Part print with two shaded views. Sizes in mm from the minimum x, y, z corner. A direction names the side the tool comes from. Round coordinates to 2 decimals unless told otherwise and drop trailing zeros. Loops run counter-clockwise (first coordinate to the right, second up) from the corner with the lowest first, then second, coordinate; pieces in that order, holes last. Notation, with made-up numbers: M 80,7.5 L 87,7.5 A20 cw 87,39.5 Z; hole C -39.5,10.5 d8. An arc over 180 degrees is marked long. Answer as CSV lines item,"result". Start each with the question number.
Item 1: Drop flat-ended pins along their axis: pin 1 Ø0.7 at (y, z) = (6.5, 2) entering from -X; pin 2 Ø3 at (x, z) = (4.5, 5.5) entering from -Y; pin 3 Ø0.8 at (x, y) = (11.5, 0.5) entering from +Z. Give the stop position or say it passes through.
Item 2: Band-saw the part on A-A (x = 12.25). Give the cut face in (y, z), and give its area (3 significant figures).
Item 3: Which spindle directions (+Z, -Z, +X, -X, +Y, -Y) get a long thin tool onto all of the face, cutting with end or side? Do the marked faces 1, 2 and 3. Say none if no direction does.
Item 4: Band-saw the part on C-C (z = 2.5). Give the cut face in (x, y), and give its area (3 significant figures).
Item 5: Band-saw the part on D-D (x = 1.65). Give the cut face in (y, z), and give its area (3 significant figures).
Item 6: Band-saw the part on B-B (y = 4.5). Give the cut face in (x, z), and give its area (3 significant figures).
Item 7: Wall check: line 1 (Y direction, x = 5.25, z = 1.75); line 2 (X direction, y = 1.5, z = 1); line 3 (X direction, y = 5.25, z = 4) (3 decimals). Give the ranges that are in metal, low to high.
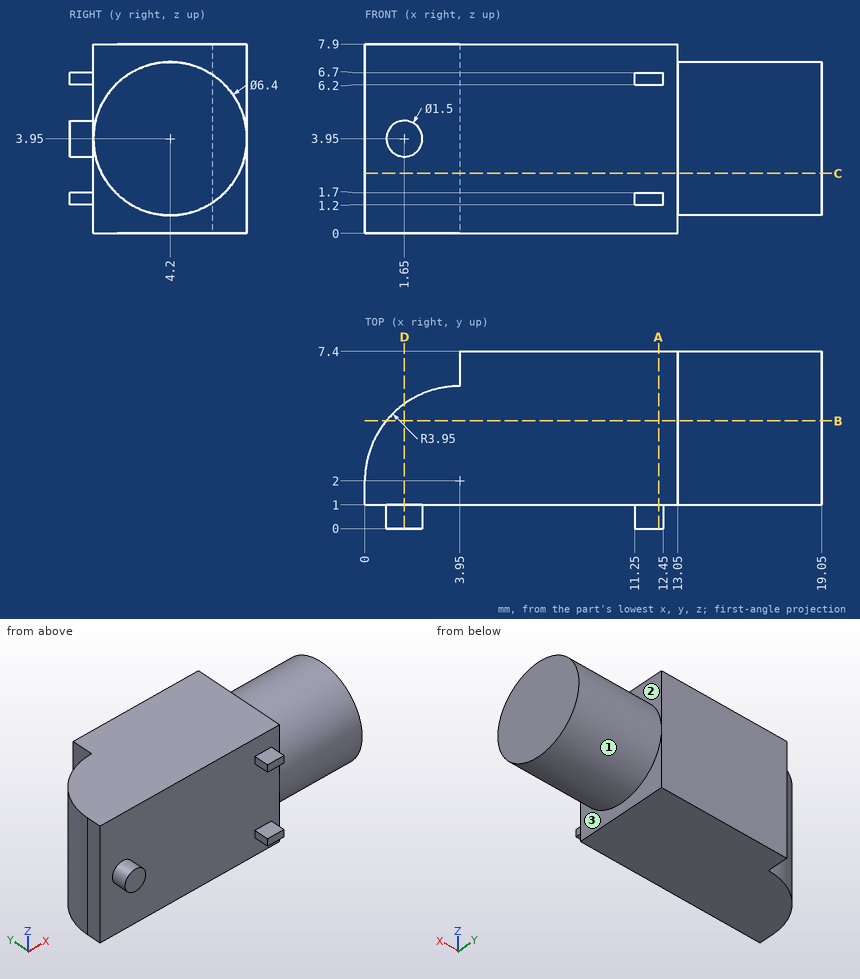
Answer block:
1,pin 1,"stops at x = 3.95"
1,pin 2,"stops at y = 1"
1,pin 3,"stops at z = 6.7"
2,outline,"M 0,1.2 L 1,1.2 L 1,0 L 7.4,0 L 7.4,7.9 L 1,7.9 L 1,6.7 L 0,6.7 L 0,6.2 L 1,6.2 L 1,1.7 L 0,1.7 Z"
2,area,"51.6 mm^2"
3,face 1,"+X"
3,face 2,"+Z, +X"
3,face 3,"-Z, +X"
4,outline,"M 0,1 L 13.05,1 L 13.05,1.35 L 19.05,1.35 L 19.05,7.05 L 13.05,7.05 L 13.05,7.4 L 3.95,7.4 L 3.95,5.95 A3.95 ccw 0,2 Z"
4,area,"109 mm^2"
5,outline,"M 0,3.2 L 1,3.2 L 1,0 L 5.21,0 L 5.21,7.9 L 1,7.9 L 1,4.7 L 0,4.7 Z"
5,area,"34.8 mm^2"
6,outline,"M 0.89,0 L 13.05,0 L 13.05,0.76 L 19.05,0.76 L 19.05,7.14 L 13.05,7.14 L 13.05,7.9 L 0.89,7.9 Z"
6,area,"134 mm^2"
7,line 1,"y = 1 to 7.4"
7,line 2,"x = 0 to 13.05"
7,line 3,"x = 1.705 to 19.05"
